```python
from build123d import *

# Parameters (mm, degrees)
SKETCH2_W                   = 77.55
SKETCH2_H                   = 12.7
F_12_0_189_DIAMETER_HOLE1_D = 4.8006
CIRPATTERN3_COUNT           = 4
CUT_EXTRUDE1_DEPTH          = 13.7
FILLET1_R                   = 4
CIRPATTERN4_COUNT           = 8
FILLET1_OF_CIRPATTERN4_R    = 4
CHAMFER1_SIZE               = 1
SKETCH15_W                  = 2.0447
SKETCH15_H                  = 101.323957926
SKETCH19_R                  = 6.25
CUT_EXTRUDE3_DEPTH          = 5
CIRPATTERN5_COUNT           = 2
CIRPATTERN6_COUNT           = 2
SKETCH22_R                  = 4.765
CUT_EXTRUDE4_DEPTH          = 12.8


with BuildPart() as part:
    # Sketch2 → Revolve1 (revolve)
    with BuildSketch(Plane(origin=(0, 0, 0), x_dir=(0, 0, -1), z_dir=(1, 0, 0))):
        with Locations((-38.775, 6.35)):
            Rectangle(SKETCH2_W, SKETCH2_H)
    revolve(axis=Axis((0, -0.888756804, 0), (0, 1, 0)))

    # #12 (0.189) Diameter Hole1 (through all)
    with Locations(Plane(origin=(0, 12.7, 0), x_dir=(1, 0, 0), z_dir=(0, 1, 0))):
        with Locations((-25.333643223, 61.160825052)):
            f_12_0_189_diameter_hole1 = Hole(F_12_0_189_DIAMETER_HOLE1_D / 2)

    # CirPattern3: #12 (0.189) Diameter Hole1 ×4 about axis
    cirpattern3_axis = Axis((0, 0, 0), (0, 1, 0))
    for i in range(1, CIRPATTERN3_COUNT):
        add(f_12_0_189_diameter_hole1.rotate(cirpattern3_axis, i * 360 / CIRPATTERN3_COUNT), mode=Mode.SUBTRACT)

    # Sketch8 → Cut-Extrude1 (cut, through all)
    with BuildSketch(Plane(origin=(0, 12.7, 0), x_dir=(1, 0, 0), z_dir=(0, 1, 0))):
        with BuildLine():
            Line((-17.167098173, 54.510670885), (-21.735525784, 65.539830782))
            ThreePointArc((-21.735525784, 65.539830782), (0, 69.05), (21.735525784, 65.539830782))
            Line((21.735525784, 65.539830782), (17.167098173, 54.510670885))
            ThreePointArc((17.167098173, 54.510670885), (0, 57.15), (-17.167098173, 54.510670885))
        make_face()
    cut_extrude1 = extrude(amount=-CUT_EXTRUDE1_DEPTH, mode=Mode.SUBTRACT)

    # Fillet1
    fillet1_edges = [part.edges().sort_by_distance(p)[0] for p in [
        (17.167098173, 6.35, -54.510670885),
        (-17.167098173, 6.35, -54.510670885),
        (-21.735525784, 6.35, -65.539830782),
        (21.735525784, 6.35, -65.539830782),
    ]]
    fillet(fillet1_edges, radius=FILLET1_R)

    # CirPattern4: Cut-Extrude1 ×8 about axis
    cirpattern4_axis = Axis((0, 0, 0), (0, 1, 0))
    for i in range(1, CIRPATTERN4_COUNT):
        add(cut_extrude1.rotate(cirpattern4_axis, i * 360 / CIRPATTERN4_COUNT), mode=Mode.SUBTRACT)

    # Fillet1 of CirPattern4
    fillet1_of_cirpattern4_edges = [part.edges().sort_by_distance(p)[0] for p in [
        (-26.405893498, 6.35, -50.683836561),
        (-50.683836561, 6.35, -26.405893498),
        (-61.712996458, 6.35, -30.974321109),
        (-30.974321109, 6.35, -61.712996458),
        (-54.510670885, 6.35, -17.167098173),
        (-54.510670885, 6.35, 17.167098173),
        (-65.539830782, 6.35, 21.735525784),
        (-65.539830782, 6.35, -21.735525784),
        (-50.683836561, 6.35, 26.405893498),
        (-26.405893498, 6.35, 50.683836561),
        (-30.974321109, 6.35, 61.712996458),
        (-61.712996458, 6.35, 30.974321109),
        (-17.167098173, 6.35, 54.510670885),
        (17.167098173, 6.35, 54.510670885),
        (21.735525784, 6.35, 65.539830782),
        (-21.735525784, 6.35, 65.539830782),
        (26.405893498, 6.35, 50.683836561),
        (50.683836561, 6.35, 26.405893498),
        (61.712996458, 6.35, 30.974321109),
        (30.974321109, 6.35, 61.712996458),
        (54.510670885, 6.35, 17.167098173),
        (54.510670885, 6.35, -17.167098173),
        (65.539830782, 6.35, -21.735525784),
        (65.539830782, 6.35, 21.735525784),
        (50.683836561, 6.35, -26.405893498),
        (26.405893498, 6.35, -50.683836561),
        (30.974321109, 6.35, -61.712996458),
        (61.712996458, 6.35, -30.974321109),
    ]]
    fillet(fillet1_of_cirpattern4_edges, radius=FILLET1_OF_CIRPATTERN4_R)

    # Chamfer1
    chamfer1_edges = [part.edges().sort_by_distance(p)[0] for p in [
        (0, 12.7, -77.55),
        (0, 0, -77.55),
    ]]
    chamfer(chamfer1_edges, length=CHAMFER1_SIZE)

    # Sketch15 → #20 (0.161) Diameter Hole1 (revolve, cut)
    with BuildSketch(Plane(origin=(0, 6.35, 0), x_dir=(-0.382683432, 0, 0.923879533), z_dir=(0, 1, 0))):
        with Locations((1.02235, 50.661978963)):
            Rectangle(SKETCH15_W, SKETCH15_H)
    revolve(axis=Axis((-5.866635031, 6.35, -2.430039796), (0.923879533, 0, 0.382683432)), mode=Mode.SUBTRACT)

    # Sketch19 → Cut-Extrude3 (cut)
    with BuildSketch(Plane(origin=(29.67710018, 0, -71.646857746), x_dir=(-0.923879533, 0, -0.382683432), z_dir=(0.382683432, 0, -0.923879533))):
        with Locations((0, 6.35)):
            Circle(SKETCH19_R)
    cut_extrude3 = extrude(amount=-CUT_EXTRUDE3_DEPTH, mode=Mode.SUBTRACT)

    # CirPattern5: Cut-Extrude3 ×2 about axis
    cirpattern5_axis = Axis((0, -0.888756804, 0), (0, 1, 0))
    for i in range(1, CIRPATTERN5_COUNT):
        add(cut_extrude3.rotate(cirpattern5_axis, i * 360 / CIRPATTERN5_COUNT), mode=Mode.SUBTRACT)

    # Sketch21 → #10-24 Tapped Hole1 (revolve, cut)
    with BuildSketch(Plane(origin=(-27.763683018, 6.35, 67.027460084), x_dir=(0.923879533, 0, 0.382683432), z_dir=(0, 1, 0))):
        Polygon((0, 0), (0, 51.940824014), (1.89865, 50.8), (1.89865, 0), align=None)
    f_10_24_tapped_hole1 = revolve(axis=Axis((-30.193722814, 6.35, 72.894095115), (0.382683432, 0, -0.923879533)), mode=Mode.SUBTRACT)

    # CirPattern6: #10-24 Tapped Hole1 ×2 about axis
    cirpattern6_axis = Axis((0, -0.888756804, 0), (0, 1, 0))
    for i in range(1, CIRPATTERN6_COUNT):
        add(f_10_24_tapped_hole1.rotate(cirpattern6_axis, i * 360 / CIRPATTERN6_COUNT), mode=Mode.SUBTRACT)

    # Sketch22 → Cut-Extrude4 (cut)
    with BuildSketch(Plane(origin=(0, 12.7, 0), x_dir=(1, 0, 0), z_dir=(0, 1, 0))):
        Circle(SKETCH22_R)
    extrude(amount=-CUT_EXTRUDE4_DEPTH, mode=Mode.SUBTRACT)


solid = part.part
```
The model under review builds one solid part; all positions refer to its coordinate system, in mm. A direction names the side the tool comes from. Round coordinates to 2 decimals unless told otherwise and drop trailing zeros.
Item 1: Machinability: for faces 5 (the conical face through (7.7, 6.3, -19.3)), 6 (the conical face through (3.373, 0.174, -76.649)), 7 (the cylindrical face through (40.55, 6.44, -40.27)), which of the approach directions +Z, -Z, +X, -X, +Y, -Y give a long, thin tool a straight path to every point of the face, cutting with its end or side? Answer none if there is none.
Working result:
face 5: none
face 6: -Y
face 7: +Y, -Y
Item 2: To check wall thickness, follow probe 1 along X at (y, z) = (7.5, 0) (3 decimals); probe 2 along X at (y, z) = (9, -18.5); probe 3 along X at (y, z) = (0.5, 53). State the ranges of each line that lie inside material, in increasing order.
Working result:
probe 1: x = -77.55 to -69.05, -57.15 to -4.765, 4.765 to 57.15, 69.05 to 77.55
probe 2: x = -75.31 to -66.33, -57.73 to 57.73, 66.33 to 75.31
probe 3: x = -55.93 to -44.26, -27.5 to 27.5, 44.26 to 55.93
Item 3: Draft analysis for pull direction Y (two halves, no side actions). For faces 1 (the conical face through (-7.7, 6.3, 19.3)), 2 (the flat face through (-29.13, 7.83, 66.46)), 3 (the conical face through (51.84, 12.54, -56.54)), 4 (the cylindrical face through (-55.73, 6.26, 16.59)), state which applies: released by +Y, released by -Y, zero draft, split by the parting line, or undercut.
Working result:
face 1: undercut
face 2: undercut
face 3: released by +Y
face 4: zero draft
Item 4: Add section A-A, the plane z = 45. Count the separate pieces of the cut face and the enclosed holes in it, and give its area (3 significant figures).
Working result:
separate pieces: 3
enclosed holes: 1
area: 1,150 mm2
Item 5: For pin 1 (1.5 mm diameter, centred on y = 9, z = -35.5, fed in from +X); pin 2 (1.5 mm diameter, centred on x = -52, y = 5.5, fed in from +Z); pin 3 (8.5 mm diameter, centred on x = 0, z = 0, fed in from +Y) (1 decimal); pin 4 (5 mm diameter, centred on x = 38.5, y = 9, fed in from +Z), all flat-tipped, find the tip position at first contact; note any pin that passes through.
Working result:
pin 1: stops at x = 69.33
pin 2: stops at z = 58.2
pin 3: passes through
pin 4: stops at z = 68.69
